Design review of the part built by this model. Coordinates are the model's own, in mm. A direction names the side the tool comes from. Coordinates: 2 decimals unless noted, no trailing zeros. Loops run counter-clockwise (first coordinate to the right, second up) from the corner with the lowest first, then second, coordinate; pieces in that order, holes last. Notation, with made-up numbers: M 14,16 L 23,16 A26 cw 23,52 Z; hole C -32.75,84 d4. An arc over 180 degrees is marked long. Answer as CSV lines item,"result". Start each with the question number.
from build123d import *

# Parameters (mm, degrees)
SKETCH_W       = 34
SKETCH_H       = 34
PAD_DEPTH      = 400
SKETCH001_R    = 5
HOLE_DEPTH     = 40.001
SKETCH002_R    = 1.75
HOLE001_DEPTH  = 40.001
SKETCH003_R    = 2
HOLE002_DEPTH  = 25
HOLE002_TIPS_R = 2
SKETCH004_W    = 25
SKETCH004_H    = 25
POCKET_DEPTH   = 3


with BuildPart() as part:
    # Sketch → Pad (new body)
    with BuildSketch(Plane.XZ):
        with BuildLine():
            Line((2, 0), (38, 0))
            ThreePointArc((38, 0), (39.414214, 0.585786), (40, 2))
            Line((40, 2), (40, 38))
            ThreePointArc((40, 38), (39.414214, 39.414214), (38, 40))
            Line((38, 40), (2, 40))
            ThreePointArc((2, 40), (0.585786, 39.414214), (0, 38))
            Line((0, 38), (0, 2))
            ThreePointArc((0, 2), (0.585786, 0.585786), (2, 0))
        make_face()
        with Locations((20, 20)):
            Rectangle(SKETCH_W, SKETCH_H, mode=Mode.SUBTRACT)
    extrude(amount=PAD_DEPTH)

    # Sketch001 (on Face5 of Pad) → Hole (cut, through all)
    with BuildSketch(Plane(origin=(0, 0, 40), x_dir=(-1, 0, 0), z_dir=(0, 0, 1))):
        with Locations((-20, 200)):
            Circle(SKETCH001_R)
    extrude(amount=-HOLE_DEPTH, mode=Mode.SUBTRACT)

    # Sketch002 (on Face10 of Hole) → Hole001 (cut, through all)
    with BuildSketch(Plane(origin=(0, 0, 40), x_dir=(-1, 0, 0), z_dir=(0, 0, 1))):
        with Locations((-12.000042, 200.025804)):
            Circle(SKETCH002_R)
        with Locations((-27.999958, 200.025804)):
            Circle(SKETCH002_R)
        with Locations((-20, 192)):
            Circle(SKETCH002_R)
        with Locations((-20, 208)):
            Circle(SKETCH002_R)
    extrude(amount=-HOLE001_DEPTH, mode=Mode.SUBTRACT)

    # Sketch003 (on Face12 of Hole001) → Hole002 (cut)
    with BuildSketch(Plane(origin=(40, 0, 0), x_dir=(0, 0, 1), z_dir=(1, 0, 0))):
        with Locations((27.886159, 10)):
            Circle(SKETCH003_R)
        with Locations((11.886159, 10)):
            Circle(SKETCH003_R)
        with Locations((27.886159, 25)):
            Circle(SKETCH003_R)
        with Locations((11.886159, 24.829785)):
            Circle(SKETCH003_R)
        with Locations((27.886159, 390)):
            Circle(SKETCH003_R)
        with Locations((11.886159, 390)):
            Circle(SKETCH003_R)
        with Locations((27.886159, 375)):
            Circle(SKETCH003_R)
        with Locations((11.886159, 375.170215)):
            Circle(SKETCH003_R)
    extrude(amount=-HOLE002_DEPTH, mode=Mode.SUBTRACT)

    # Hole002 tips → Hole002 tip 1 section 0
    with BuildSketch(Plane(origin=(15, 0, 0), x_dir=(0, 0, 1), z_dir=(1, 0, 0)), mode=Mode.PRIVATE) as hole002_tip_1_s0:
        with Locations((27.886159, 10)):
            Circle(HOLE002_TIPS_R)
    loft([hole002_tip_1_s0.sketch, Vertex(13.798279, -10, 27.886159)], mode=Mode.SUBTRACT)

    # Hole002 tips → Hole002 tip 2 section 0
    with BuildSketch(Plane(origin=(15, 0, 0), x_dir=(0, 0, 1), z_dir=(1, 0, 0)), mode=Mode.PRIVATE) as hole002_tip_2_s0:
        with Locations((11.886159, 10)):
            Circle(HOLE002_TIPS_R)
    loft([hole002_tip_2_s0.sketch, Vertex(13.798279, -10, 11.886159)], mode=Mode.SUBTRACT)

    # Hole002 tips → Hole002 tip 3 section 0
    with BuildSketch(Plane(origin=(15, 0, 0), x_dir=(0, 0, 1), z_dir=(1, 0, 0)), mode=Mode.PRIVATE) as hole002_tip_3_s0:
        with Locations((27.886159, 25)):
            Circle(HOLE002_TIPS_R)
    loft([hole002_tip_3_s0.sketch, Vertex(13.798279, -25, 27.886159)], mode=Mode.SUBTRACT)

    # Hole002 tips → Hole002 tip 4 section 0
    with BuildSketch(Plane(origin=(15, 0, 0), x_dir=(0, 0, 1), z_dir=(1, 0, 0)), mode=Mode.PRIVATE) as hole002_tip_4_s0:
        with Locations((11.886159, 24.829785)):
            Circle(HOLE002_TIPS_R)
    loft([hole002_tip_4_s0.sketch, Vertex(13.798279, -24.829785, 11.886159)], mode=Mode.SUBTRACT)

    # Hole002 tips → Hole002 tip 5 section 0
    with BuildSketch(Plane(origin=(15, 0, 0), x_dir=(0, 0, 1), z_dir=(1, 0, 0)), mode=Mode.PRIVATE) as hole002_tip_5_s0:
        with Locations((27.886159, 390)):
            Circle(HOLE002_TIPS_R)
    loft([hole002_tip_5_s0.sketch, Vertex(13.798279, -390, 27.886159)], mode=Mode.SUBTRACT)

    # Hole002 tips → Hole002 tip 6 section 0
    with BuildSketch(Plane(origin=(15, 0, 0), x_dir=(0, 0, 1), z_dir=(1, 0, 0)), mode=Mode.PRIVATE) as hole002_tip_6_s0:
        with Locations((11.886159, 390)):
            Circle(HOLE002_TIPS_R)
    loft([hole002_tip_6_s0.sketch, Vertex(13.798279, -390, 11.886159)], mode=Mode.SUBTRACT)

    # Hole002 tips → Hole002 tip 7 section 0
    with BuildSketch(Plane(origin=(15, 0, 0), x_dir=(0, 0, 1), z_dir=(1, 0, 0)), mode=Mode.PRIVATE) as hole002_tip_7_s0:
        with Locations((27.886159, 375)):
            Circle(HOLE002_TIPS_R)
    loft([hole002_tip_7_s0.sketch, Vertex(13.798279, -375, 27.886159)], mode=Mode.SUBTRACT)

    # Hole002 tips → Hole002 tip 8 section 0
    with BuildSketch(Plane(origin=(15, 0, 0), x_dir=(0, 0, 1), z_dir=(1, 0, 0)), mode=Mode.PRIVATE) as hole002_tip_8_s0:
        with Locations((11.886159, 375.170215)):
            Circle(HOLE002_TIPS_R)
    loft([hole002_tip_8_s0.sketch, Vertex(13.798279, -375.170215, 11.886159)], mode=Mode.SUBTRACT)

    # Sketch004 (on Face11 of Hole002) → Pocket (cut)
    with BuildSketch(Plane(origin=(0, 0, 0), x_dir=(0, 0, -1), z_dir=(-1, 0, 0))):
        with Locations((-20, 17.5)):
            Rectangle(SKETCH004_W, SKETCH004_H)
        with Locations((-20, 382.5)):
            Rectangle(SKETCH004_W, SKETCH004_H)
    extrude(amount=-POCKET_DEPTH, mode=Mode.SUBTRACT)


solid = part.part
Item 1: Add section B-B (x = 33). Give the boundary of the cut face in (y, z).
Item 2: For faces 4 (the face through (27, -197, 37)), 5 (the face through (20.651, -204.957, 1.521)), list the 3-axis set-ups (+Z, -Z, +X, -X, +Y, -Y) from which the entire face can be reached by the end or side of a thin tool; tool diameter is ignored.
Item 3: Add section A-A (y = -47). Give the boundary of the cut face in (x, z), plus the area to 3 significant figures.
Item 4: For pin 1 (3.5 mm diameter, centred on x = 1.5, y = -376.5, fed in from -Z); pin 2 (5 mm diameter, centred on y = -375, z = 27.89, fed in from -X), all flat-tipped, find the tip position at first contact; note any pin that passes through.
Item 5: For line 1 along Y through (x, z) = (20, 0.9); line 2 along Z through (x, y) = (38, -390); line 3 along X through (y, z) = (-168, 36.5), list the stretches that pass through material, from the lowest coordinate up. Write a range as from..to.
Item 6: Mouldability with a two-part tool opening along X and no side actions: class faces 1 (the face through (40, -197, 20)), 2 (the face through (28, -197, 40)), 3 (the face through (27, -197, 3)) as released by +X, released by -X, zero draft, split by the parting line, or undercut.
Response:
1,outline,"M -400,0 L 0,0 L 0,3 L -400,3 Z; M -400,37 L 0,37 L 0,40 L -400,40 Z"
2,face 4,"+Y, -Y"
2,face 5,"+Z, -Z"
3,outline,"M 0,2 A2 ccw 2,0 L 38,0 A2 ccw 40,2 L 40,38 A2 ccw 38,40 L 2,40 A2 ccw 0,38 Z; hole M 3,3 L 37,3 L 37,37 L 3,37 Z"
3,area,"441 mm²"
4,pin 1,"z = 0"
4,pin 2,"x = 37"
5,line 1,"-400..-209.75, -206.25..-205, -195..-193.75, -190.25..0"
5,line 2,"0..9.89, 13.89..25.89, 29.89..40"
5,line 3,"0..3, 37..40"
6,face 1,"released by +X"
6,face 2,"zero draft"
6,face 3,"undercut"
